Print and shaded views of the part. All mm, measured from the part's lowest x, y and z. A direction names the side the tool comes from. Coordinates: 2 decimals unless noted, no trailing zeros. Order: outer loops, then holes, each group sorted by start corner. A loop starts at its lowest first (then second) coordinate and runs counter-clockwise, first axis right, second up.
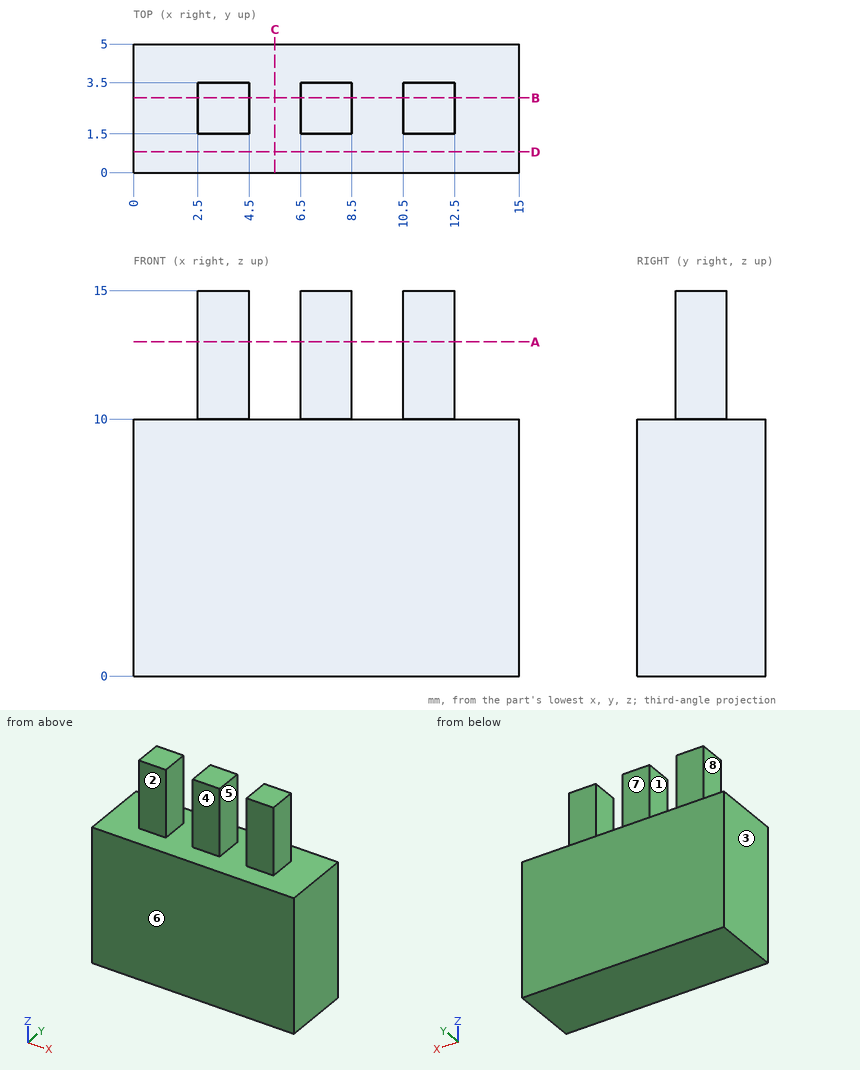
Q1. Cut at C-C, the plane x = 5.5. List the corners of the cut face in (y, z), plus the area to 3 significant figures.
Established:
outline: (0, 0) - (5, 0) - (5, 10) - (0, 10) - close
area: 50.0 mm2
Q2. Cut at D-D, the plane y = 0.8. List the corners of the cut face in (x, z).
Established:
outline: (0, 0) - (15, 0) - (15, 10) - (0, 10) - close
Q3. Mould opens along X. For the marked faces 1, 2 and 3 say: pulls with the +X half, pulls with the -X half, needs draft (parallel to the pull), parting line crosses it, or undercut.
Established:
face 1: undercut
face 2: needs draft
face 3: pulls with the -X half
Q4. Cut at A-A, the plane z = 13. List the corners of the cut face in (x, y), plus the area to 3 significant figures.
Established:
outline: (2.5, 1.5) - (4.5, 1.5) - (4.5, 3.5) - (2.5, 3.5) - close; (6.5, 1.5) - (8.5, 1.5) - (8.5, 3.5) - (6.5, 3.5) - close; (10.5, 1.5) - (12.5, 1.5) - (12.5, 3.5) - (10.5, 3.5) - close
area: 12.0 mm2
Q5. Drop flat-ended pins along their axis: P1, Ø2, axis at x = 3.5, z = 12.5, coming from the -Y side; P2, Ø2, axis at y = 2.5, z = 11.5, coming from the -X side; P3, Ø5, axis at x = 12.5, z = 7, coming from the -Y side; P4, Ø1.6, axis at x = 8, z = 12.5, coming from the +Y side. Give the stop position or say it passes through.
Established:
P1: stops at y = 1.5
P2: stops at x = 2.5
P3: stops at y = 0
P4: stops at y = 3.5
Q6. Which spindle directions (+Z, -Z, +X, -X, +Y, -Y) get a long thin tool onto all of the face, cutting with end or side? Do the marked faces 4, 5, 6, 7 and 8. Say none if no direction does.
Established:
face 4: +Z, +X, -X, -Y
face 5: +Z, +Y, -Y
face 6: +Z, -Z, +X, -X, -Y
face 7: +Z, +X, -X, +Y
face 8: +Z, -X, +Y, -Y
Q7. Cut at B-B, the plane y = 2.9. List the corners of the cut face in (x, z), plus the area to 3 significant figures.
Established:
outline: (0, 0) - (15, 0) - (15, 10) - (12.5, 10) - (12.5, 15) - (10.5, 15) - (10.5, 10) - (8.5, 10) - (8.5, 15) - (6.5, 15) - (6.5, 10) - (4.5, 10) - (4.5, 15) - (2.5, 15) - (2.5, 10) - (0, 10) - close
area: 180 mm2
Q8. Probe line 1 (X direction, y = 2.2, z = 10.25); line 2 (Z direction, x = 7.5, y = 1.45). List the from-to ranges inside material, lowest first.
Established:
line 1: x = 2.5 to 4.5, 6.5 to 8.5, 10.5 to 12.5
line 2: z = 0 to 10
